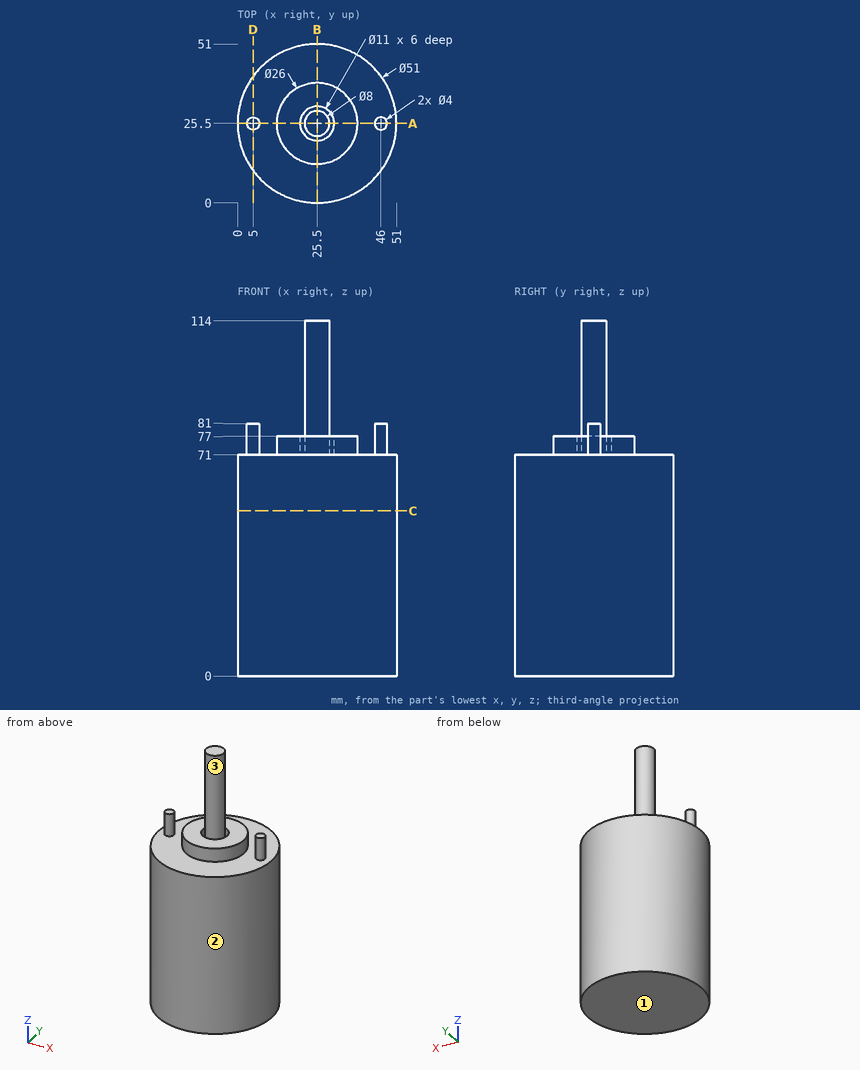
Geometry check sheet. Reference: drawing and pictorial views, mm from the part's lowest x, y, z. Round coordinates to 2 decimals unless told otherwise and drop trailing zeros. Order: outer loops, then holes, each group sorted by start corner. A loop starts at its lowest first (then second) coordinate and runs counter-clockwise, first axis right, second up. Notation, with made-up numbers: M -19,48 L 21,48 A15 cw 21,52 Z; hole C -26,58 d2. An arc over 180 degrees is marked long. One line per item, written item: value. Start each with the question number.
1. Section check B-B on x = 25.5. Enter the section's corners in (y, z), and give its area (4 significant figures).
2. Section check D-D on x = 5. Enter the section's corners in (y, z), and give its area (3 significant figures).
3. Scan lines: line 1 along Y through (x, z) = (25.5, 73.25); line 2 along X through (y, z) = (25, 73); line 3 along Z through (x, y) = (4.5, 19). Record each from-to range of solid material in increasing order.
4. Release check for a two-part mould opening along X. For the marked faces 1, 2 and 3 record: released by +X, released by -X, zero draft, split by the parting line, or undercut.
5. Section check C-C on z = 53. Enter the section's corners in (x, y), and give its area (3 significant figures).
6. Gauge pin test, flat ends, axial feed: P1, Ø5, axis at x = 23.5, z = 25, coming from the +Y side; P2, Ø2, axis at x = 6.5, y = 26, coming from the +Z side; P3, Ø12, axis at y = 18.5, z = 66.5, coming from the -X side. Record the tip position at first contact, or that the pin passes through.
7. Section check A-A on y = 25.5. Enter the section's corners in (x, z).
Results found:
1. outline: M 0,0 L 51,0 L 51,71 L 38.5,71 L 38.5,77 L 31,77 L 31,71 L 29.5,71 L 29.5,114 L 21.5,114 L 21.5,71 L 20,71 L 20,77 L 12.5,77 L 12.5,71 L 0,71 Z
1. area: 4,055 mm^2
2. outline: M 10.33,0 L 40.67,0 L 40.67,71 L 27.5,71 L 27.5,81 L 23.5,81 L 23.5,71 L 10.33,71 Z
2. area: 2,190 mm^2
3. line 1: 12.5 to 20, 21.5 to 29.5, 31 to 38.5
3. line 2: 3.06 to 6.94, 12.51 to 20.02, 21.53 to 29.47, 30.98 to 38.49, 44.06 to 47.94
3. line 3: 0 to 71
4. face 1: zero draft
4. face 2: split by the parting line
4. face 3: undercut
5. outline: C 25.5,25.5 d51
5. area: 2,040 mm^2
6. P1: y = 51
6. P2: z = 81
6. P3: x = 0.02
7. outline: M 0,0 L 51,0 L 51,71 L 48,71 L 48,81 L 44,81 L 44,71 L 38.5,71 L 38.5,77 L 31,77 L 31,71 L 29.5,71 L 29.5,114 L 21.5,114 L 21.5,71 L 20,71 L 20,77 L 12.5,77 L 12.5,71 L 7,71 L 7,81 L 3,81 L 3,71 L 0,71 Z
